Design review of the part built by this model. Coordinates are the model's own, in mm. A direction names the side the tool comes from. Give positions to 0.01 mm unless a question says otherwise; leave off trailing zeros. Write each loop counter-clockwise with the first axis right and the second up, starting at its lowest first coordinate (ties: lowest second). Pieces come first, ordered by that corner, then holes. Notation, with made-up numbers: M 45.25,82 L 96.25,82 A10 ccw 96.25,99 Z; hole C 83.5,31.25 d11. An arc over 180 degrees is marked long. Use one line per item in the form item = value. Start each with the question number.
from build123d import *

# Parameters (mm, degrees)
EXTRUDE1_DEPTH = 324
SKETCH2_R      = 2.5
EXTRUDE2_DEPTH = 36
EXTRUDE3_DEPTH = 17
SKETCH4_R      = 2.5
EXTRUDE4_DEPTH = 97


with BuildPart() as part:
    # Sketch1 → Extrude1 (new body)
    with BuildSketch(Plane.XY):
        with BuildLine():
            Line((-17.939611789, -4.078161588), (13.060388211, -4.078161588))
            ThreePointArc((13.060388211, -4.078161588), (14.474601773, -4.663948025), (15.060388211, -6.078161588))
            Line((15.060388211, -6.078161588), (15.060388211, -60.078161588))
            ThreePointArc((15.060388211, -60.078161588), (14.474601773, -61.49237515), (13.060388211, -62.078161588))
            Line((13.060388211, -62.078161588), (-17.939611789, -62.078161588))
            ThreePointArc((-17.939611789, -62.078161588), (-19.353825352, -61.49237515), (-19.939611789, -60.078161588))
            Line((-19.939611789, -60.078161588), (-19.939611789, -6.078161588))
            ThreePointArc((-19.939611789, -6.078161588), (-19.353825352, -4.663948025), (-17.939611789, -4.078161588))
        make_face()
        with BuildLine():
            Line((-15.939611789, -6.078161588), (11.060388211, -6.078161588))
            ThreePointArc((11.060388211, -6.078161588), (12.474601773, -6.663948025), (13.060388211, -8.078161588))
            Line((13.060388211, -8.078161588), (13.060388211, -58.078161588))
            ThreePointArc((13.060388211, -58.078161588), (12.474601773, -59.49237515), (11.060388211, -60.078161588))
            Line((11.060388211, -60.078161588), (-15.939611789, -60.078161588))
            ThreePointArc((-15.939611789, -60.078161588), (-17.353825352, -59.49237515), (-17.939611789, -58.078161588))
            Line((-17.939611789, -58.078161588), (-17.939611789, -8.078161588))
            ThreePointArc((-17.939611789, -8.078161588), (-17.353825352, -6.663948025), (-15.939611789, -6.078161588))
        make_face(mode=Mode.SUBTRACT)
    extrude(amount=EXTRUDE1_DEPTH)

    # Sketch2 → Extrude2 (cut, through all)
    with BuildSketch(Plane(origin=(15.060388211, 0, 0), x_dir=(0, 0, -1), z_dir=(1, 0, 0))):
        with Locations((-9, -54.078161588)):
            Circle(SKETCH2_R)
        with Locations((-99, -54.078161588)):
            Circle(SKETCH2_R)
        with BuildLine():
            Line((0, -44.078161588), (-43, -44.078161588))
            ThreePointArc((-43, -44.078161588), (-53.606601718, -39.684763305), (-58, -29.078161588))
            Line((-58, -29.078161588), (-58, -4.078161588))
            Line((-58, -4.078161588), (0, -4.078161588))
            Line((0, -4.078161588), (0, -44.078161588))
        make_face()
        with BuildLine():
            Line((-324, -41.078161588), (-278, -41.078161588))
            ThreePointArc((-278, -41.078161588), (-267.393398282, -36.684763305), (-263, -26.078161588))
            Line((-263, -26.078161588), (-263, -4.078161588))
            Line((-263, -4.078161588), (-324, -4.078161588))
            Line((-324, -4.078161588), (-324, -41.078161588))
        make_face()
    extrude(amount=-EXTRUDE2_DEPTH, mode=Mode.SUBTRACT)

    # Sketch3 → Extrude3 (add)
    with BuildSketch(Plane.XZ.offset(62.078161588)):
        Polygon((15.060388211, 324), (15.060388211, 289), (22.060388211, 289), (22.060388211, 324), (22.060388211, 354), (45.560388211, 410), (45.560388211, 534), (38.560388211, 534), (38.560388211, 410), (15.060388211, 354), align=None)
        Polygon((-19.939611789, 324), (-19.939611789, 289), (-26.939611789, 289), (-26.939611789, 324), (-26.939611789, 354), (-50.439611789, 410), (-50.439611789, 534), (-43.439611789, 534), (-43.439611789, 410), (-19.939611789, 354), align=None)
    extrude(amount=-EXTRUDE3_DEPTH)

    # Sketch4 → Extrude4 (cut, through all)
    with BuildSketch(Plane(origin=(45.560388211, 0, 0), x_dir=(0, 0, -1), z_dir=(1, 0, 0))):
        with Locations((-529, -54.078161588)):
            Circle(SKETCH4_R)
    extrude(amount=-EXTRUDE4_DEPTH, mode=Mode.SUBTRACT)


solid = part.part
1. We need section B-B (z = 494). State the section outline as (x, y) points, and give its area (3 significant figures).
2. We need section A-A (x = 1). State the section outline as (y, z) points.
3. To check wall thickness, follow L1, parallel to Y at x = 40, z = 529; L2, parallel to X at y = -45, z = 186; L3, parallel to X at y = -48, z = 418.5. State the ranges of each line that lie inside material, in increasing order.
4. Draft analysis for pull direction Y (two halves, no side actions). For faces 1 (the flat face through (-17.94, -39, 160)), 2 (the flat face through (-43.44, -54, 473)), 3 (the flat face through (40, -45.078, 412)), state which applies: pulls with the +Y half, pulls with the -Y half, needs draft (parallel to the pull), parting line crosses it, or undercut.
5. For faces 4 (the flat face through (38.56, -54, 473)), 5 (the flat face through (-2, -60.078, 160)), 6 (the flat face through (-26.94, -54, 322)), 7 (the flat face through (0, -5, 263)), list the 3-axis set-ups (+Z, -Z, +X, -X, +Y, -Y) from which the entire face can be reached by the end or side of a thin tool; tool diameter is ignored.
6. We need section C-C (z = 234). State the section outline as (x, y) points, and give its area (3 significant figures).
7. Clearance check with flat-ended pins moving along their axes: pin 1 Ø2 at (x, z) = (14.5, 299) entering from +Y; pin 2 Ø5.5 at (x, y) = (-23, -55) entering from -Z; pin 3 Ø15.5 at (x, z) = (35.5, 392) entering from +Y. State where each tip first meets the part, or that it passes through.
Answer block:
q1.outline = M -50.44,-62.08 L -43.44,-62.08 L -43.44,-45.08 L -50.44,-45.08 Z; M 38.56,-62.08 L 45.56,-62.08 L 45.56,-45.08 L 38.56,-45.08 Z
q1.area = 238 mm^2
q2.outline = M -62.08,0 L -60.08,0 L -60.08,324 L -62.08,324 Z; M -6.08,58 L -4.08,58 L -4.08,263 L -6.08,263 Z
q3.L1 = -62.08 to -56.58, -51.58 to -45.08
q3.L2 = -19.94 to -17.94, 13.06 to 15.06
q3.L3 = -50.44 to -43.44, 38.56 to 45.56
q4.face_1 = undercut
q4.face_2 = needs draft
q4.face_3 = pulls with the +Y half
q5.face_4 = +Z, +Y, -Y
q5.face_5 = +Z, -Z
q5.face_6 = -Z, -X, +Y, -Y
q5.face_7 = +Z, +X, -X, +Y
q6.outline = M -19.94,-60.08 A2 ccw -17.94,-62.08 L 13.06,-62.08 A2 ccw 15.06,-60.08 L 15.06,-6.08 A2 ccw 13.06,-4.08 L -17.94,-4.08 A2 ccw -19.94,-6.08 Z; hole M -17.94,-58.08 A2 ccw -15.94,-60.08 L 11.06,-60.08 A2 ccw 13.06,-58.08 L 13.06,-8.08 A2 ccw 11.06,-6.08 L -15.94,-6.08 A2 ccw -17.94,-8.08 Z
q6.area = 356 mm^2
q7.pin_1 = -41.08
q7.pin_2 = 289
q7.pin_3 = -45.08
